For this review, use the dimensioned drawing (mm, ordinates from the lowest corner) and the shaded views. A direction names the side the tool comes from. Coordinates: 2 decimals unless noted, no trailing zeros. Write each loop counter-clockwise with the first axis right and the second up, starting at its lowest first coordinate (ties: lowest second). Pieces come first, ordered by that corner, then holes. Notation, with made-up numbers: M -5.5,65 L 35.5,65 A27 cw 35.5,97 Z; hole C -31.5,-24.75 d5. An arc over 180 degrees is marked long. Return JSON: item names as keys, results as strings.
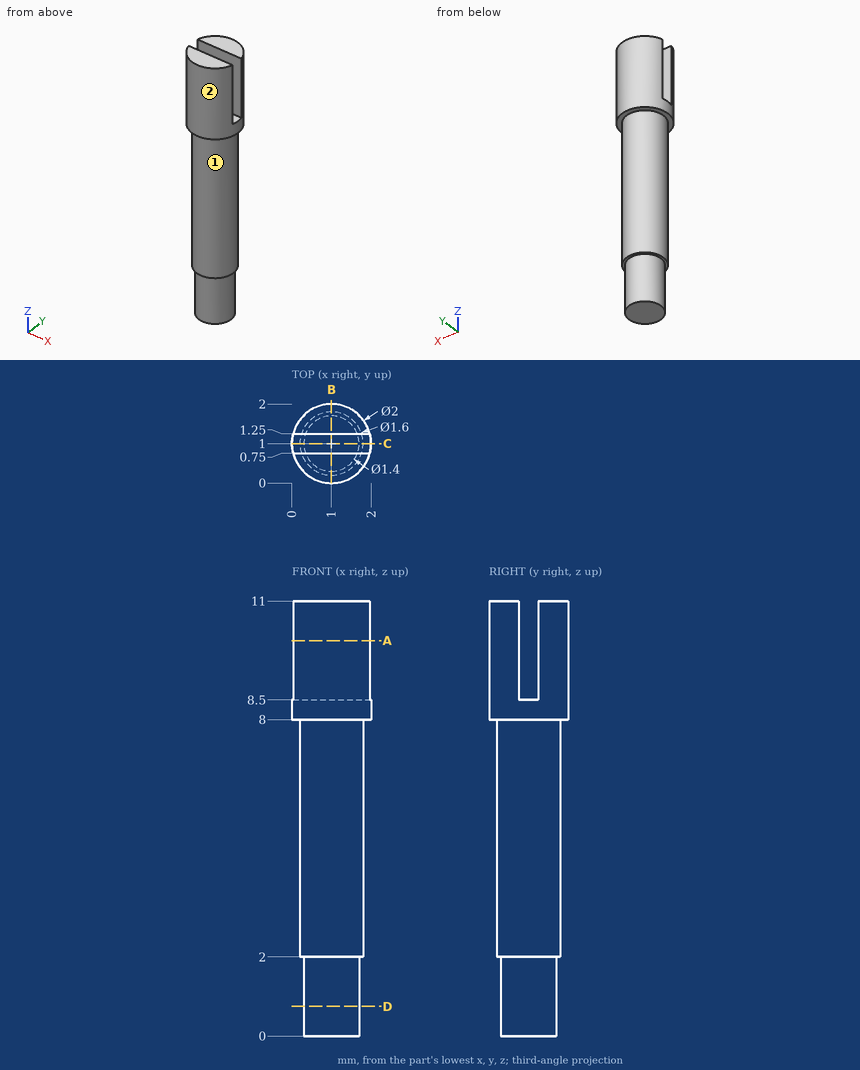
1. For the marked faces 1 and 2, list the 3-axis set-ups (+Z, -Z, +X, -X, +Y, -Y) from which the entire face can be reached by the end or side of a thin tool; tool diameter is ignored.
Checks:
{"face 1": "-Z", "face 2": "+Z, -Z"}
2. We need section A-A (z = 10). State the section outline as (x, y) points, plus the area to 3 significant figures.
Checks:
{"outline": "M 0.03,0.75 A1 ccw 1.97,0.75 Z; M 0.03,1.25 L 1.97,1.25 A1 ccw Z", "area": "2.15 mm2"}
3. Wall thickness on L1, parallel to X at y = 1, z = 4.5; L2, parallel to Z at x = 1.85, y = 1.15; L3, parallel to Z at x = 1.8, y = 1.4: over which ranges is each line inside the solid? List them lowest first. Write a range as from..to.
Checks:
{"L1": "0.2..1.8", "L2": "8..8.5", "L3": "8..11"}
4. We need section B-B (x = 1). State the section outline as (y, z) points, plus the area to 4 significant figures.
Checks:
{"outline": "M 0,8 L 0.2,8 L 0.2,2 L 0.3,2 L 0.3,0 L 1.7,0 L 1.7,2 L 1.8,2 L 1.8,8 L 2,8 L 2,11 L 1.25,11 L 1.25,8.5 L 0.75,8.5 L 0.75,11 L 0,11 Z", "area": "17.15 mm2"}
5. We need section C-C (y = 1). State the section outline as (x, z) points.
Checks:
{"outline": "M 0,8 L 0.2,8 L 0.2,2 L 0.3,2 L 0.3,0 L 1.7,0 L 1.7,2 L 1.8,2 L 1.8,8 L 2,8 L 2,8.5 L 0,8.5 Z"}
6. We need section D-D (z = 0.75). State the section outline as (x, y) points, plus the area to 3 significant figures.
Checks:
{"outline": "C 1,1 d1.4", "area": "1.54 mm2"}
